Check sheet for the modelled part. Datum: model origin and axes. Units: mm. Face numbers are marked on the shaded views. A direction names the side the tool comes from. Coordinates: 2 decimals unless noted, no trailing zeros. Order: outer loops, then holes, each group sorted by start corner. A loop starts at its lowest first (then second) coordinate and runs counter-clockwise, first axis right, second up.
1. Set-up check for the marked faces 1, 2 and 3: record each of +Z, -Z, +X, -X, +Y, -Y from which the full face is reachable in a straight line by a thin tool's end or side.
2. Cross-section at D-D (z = -14). Enter the section's corners in (x, y), then the cut area to 3 significant figures.
3. Cross-section at C-C (y = 35.5). Enter the section's corners in (x, z).
4. Draft check along X on the marked faces 4, 5 and 6. Enter one of: released by +X, released by -X, zero draft, split by the parting line, or undercut.
5. Cross-section at A-A (z = -37). Enter the section's corners in (x, y), then the cut area to 3 significant figures.
6. Gauge pin test, flat ends, axial feed: pin 1 Ø6 at (x, y) = (13, 12.5) entering from +Z; pin 2 Ø24 at (x, z) = (40, -35) entering from +Y; pin 3 Ø6 at (y, z) = (34, -31) entering from -X. Record the tip position at first contact, or that the pin passes through.
7. Cross-section at B-B (x = 42.5). Enter the section's corners in (y, z).
8. Thickness scan on line 1 (Z direction, x = 12.5, y = 15); line 2 (Z direction, x = 6, y = 22); line 3 (X direction, y = 33, z = -37). Record the ranges inside material, lowest first.
```python
from build123d import *

# Parameters (mm, degrees)
SKETCH1_W           = 80
SKETCH1_H           = 50
BOSS_EXTRUDE2_DEPTH = 50
SKETCH2_W           = 60
SKETCH2_H           = 10
CUT_EXTRUDE1_DEPTH  = 50
SKETCH3_W           = 30
SKETCH3_H           = 10
CUT_EXTRUDE2_DEPTH  = 50
CUT_EXTRUDE3_DEPTH  = 50
CUT_EXTRUDE4_DEPTH  = 20
CUT_EXTRUDE5_DEPTH  = 10


with BuildPart() as part:
    # Sketch1 → Boss-Extrude2 (new body)
    with BuildSketch(Plane.XY):
        with Locations((40, 25)):
            Rectangle(SKETCH1_W, SKETCH1_H)
    extrude(amount=-BOSS_EXTRUDE2_DEPTH)

    # Sketch2 → Cut-Extrude1 (cut)
    with BuildSketch(Plane.XY):
        with Locations((30, 45)):
            Rectangle(SKETCH2_W, SKETCH2_H)
    extrude(amount=-CUT_EXTRUDE1_DEPTH, mode=Mode.SUBTRACT)

    # Sketch3 → Cut-Extrude2 (cut)
    with BuildSketch(Plane.XY):
        with Locations((15, 35)):
            Rectangle(SKETCH3_W, SKETCH3_H)
    extrude(amount=-CUT_EXTRUDE2_DEPTH, mode=Mode.SUBTRACT)

    # Sketch4 → Cut-Extrude3 (cut)
    with BuildSketch(Plane.XZ):
        Polygon((60, 0), (0, 0), (0, -10), (50, -10), align=None)
    extrude(amount=-CUT_EXTRUDE3_DEPTH, mode=Mode.SUBTRACT)

    # Sketch5 → Cut-Extrude4 (cut)
    with BuildSketch(Plane(origin=(0, 40, 0), x_dir=(1, 0, 0), z_dir=(0, 1, 0))):
        Polygon((50, 10), (30, 30), (30, 10), align=None)
    extrude(amount=-CUT_EXTRUDE4_DEPTH, mode=Mode.SUBTRACT)

    # Sketch6 → Cut-Extrude5 (cut)
    with BuildSketch(Plane(origin=(0, 30, 0), x_dir=(1, 0, 0), z_dir=(0, 1, 0))):
        Polygon((0, 10), (50, 10), (20, 40), (0, 40), align=None)
    extrude(amount=-CUT_EXTRUDE5_DEPTH, mode=Mode.SUBTRACT)


solid = part.part
```
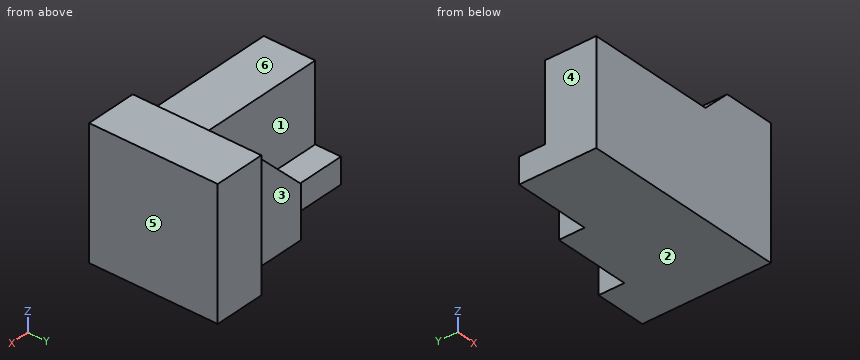
Data:
1. face 1: +Z, -X, +Y
1. face 2: -Z, +X, -X, +Y, -Y
1. face 3: +Z, -Z, -X, +Y
2. outline: (0, 0) - (80, 0) - (80, 50) - (60, 50) - (60, 40) - (46, 40) - (46, 20) - (0, 20) - close
2. area: 2,480 mm2
3. outline: (30, -50) - (80, -50) - (80, 0) - (60, 0) - (30, -30) - close
4. face 4: released by -X
4. face 5: released by +X
4. face 6: zero draft
5. outline: (0, 0) - (80, 0) - (80, 50) - (60, 50) - (60, 40) - (30, 40) - (30, 30) - (23, 30) - (23, 20) - (0, 20) - close
5. area: 2,870 mm2
6. pin 1: stops at z = -10
6. pin 2: stops at y = 40
6. pin 3: stops at x = 30
7. outline: (0, -50) - (40, -50) - (40, -17.5) - (20, -17.5) - (20, -10) - (0, -10) - close
8. line 1: z = -50 to -10
8. line 2: z = -50 to -40
8. line 3: x = 30 to 80
